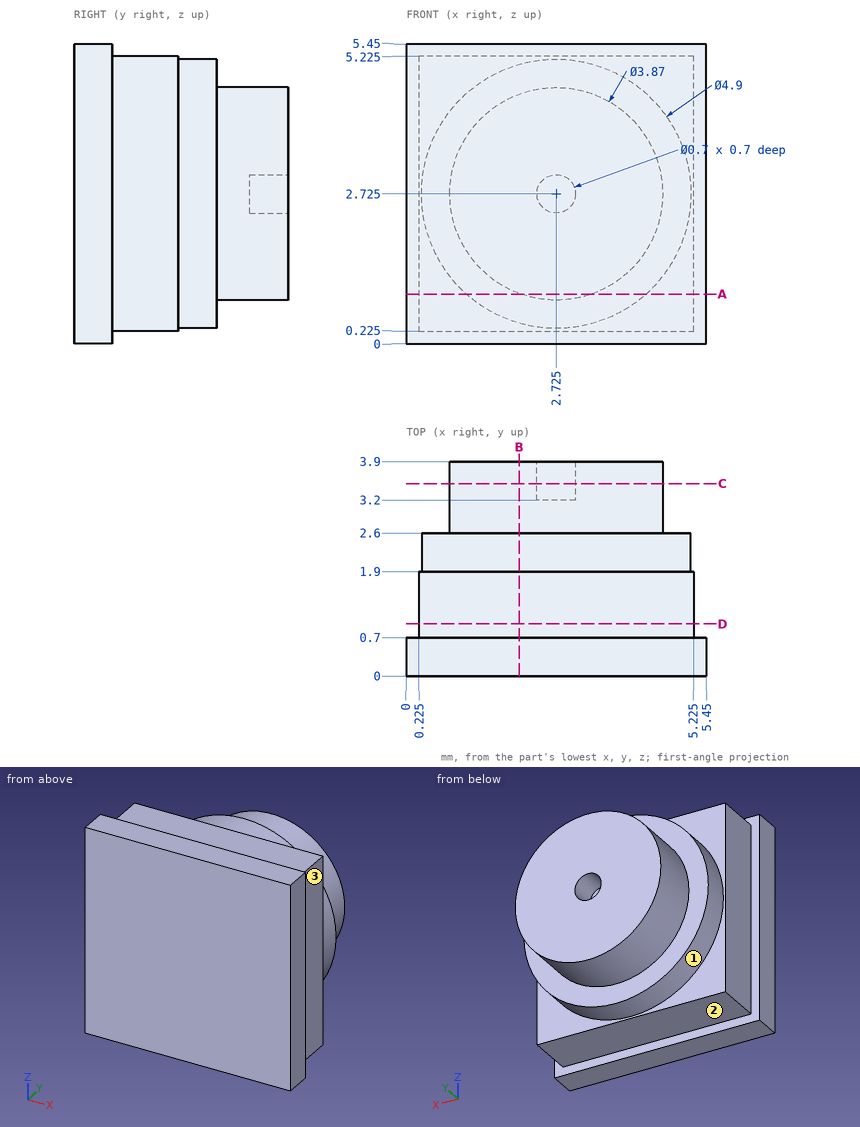
Input: dimensioned drawing with shaded views. Units: mm. Origin: part minimum x, y, z. A direction names the side the tool comes from. Give positions to 0.01 mm unless a question says otherwise; leave off trailing zeros. Order: outer loops, then holes, each group sorted by start corner. A loop starts at its lowest first (then second) coordinate and runs counter-clockwise, first axis right, second up.
(1) Section query D-D (y = 0.95). Return the cut outline in (x, z) (3 decimals).
(2) Section query B-B (x = 2.05). Return the cut outline in (y, z) (3 decimals), plus the area to 3 significant figures.
(3) Contact query for flat-ended pins moving along their axis: P1, Ø1, axis at y = 1, z = 2, coming from the -X side; P2, Ø1.5, axis at y = 2, z = 4, coming from the -X side (3 decimals); P3, Ø0.6, axis at y = 1.5, z = 3.5, coming from the +X side (3 decimals). Output: stop coordinate, or through.
(4) Section query C-C (y = 3.5). Return the cut outline in (x, z) (3 decimals).
(5) Material intervals for line 1 along X through (y, z) = (1.2, 3.8) (3 decimals); line 2 along Y through (x, z) = (2.95, 0.55), sorted ascending.
(6) Section query A-A (z = 0.9). Return the cut outline in (x, y) (3 decimals).
(7) Access query for the marked faces 1, 2 and 3. Directions: +Z, -Z, +X, -X, +Y, -Y. A direction counts if a zero-diameter tool reaches every point of the face in a straight line with its end or side. Return the directions, or none.
Outcome:
1. outline: (0.225, 0.225) - (5.225, 0.225) - (5.225, 5.225) - (0.225, 5.225) - close
2. outline: (0, 0) - (0.7, 0) - (0.7, 0.225) - (1.9, 0.225) - (1.9, 0.37) - (2.6, 0.37) - (2.6, 0.912) - (3.9, 0.912) - (3.9, 4.538) - (2.6, 4.538) - (2.6, 5.08) - (1.9, 5.08) - (1.9, 5.225) - (0.7, 5.225) - (0.7, 5.45) - (0, 5.45) - close
2. area: 17.8 mm2
3. P1: stops at x = 0
3. P2: stops at x = 0.225
3. P3: stops at x = 5.225
4. outline: circle Ø3.87 at (2.725, 2.725); hole circle Ø0.7 at (2.725, 2.725)
5. line 1: x = 0.225 to 5.225
5. line 2: y = 0 to 2.6
6. outline: (0, 0) - (5.45, 0) - (5.45, 0.7) - (5.225, 0.7) - (5.225, 1.9) - (4.36, 1.9) - (4.36, 2.6) - (3.368, 2.6) - (3.368, 3.9) - (2.082, 3.9) - (2.082, 2.6) - (1.09, 2.6) - (1.09, 1.9) - (0.225, 1.9) - (0.225, 0.7) - (0, 0.7) - close
7. face 1: +Y
7. face 2: -Z, +X, -X, +Y
7. face 3: +Z, -Z, +X, +Y
